from build123d import *

# Parameters (mm, degrees)
F0_R     = 22.03
F1_DEPTH = 50
F2_R     = 5


with BuildPart() as f1:
    # F0 (on Top) → F1 (new body)
    with BuildSketch(Plane.XY):
        with BuildLine():
            ThreePointArc((19.111431778, -6.8960115293), (56.4366245885, -5.6218490797), (74.7410013376, 26.9318496366))
            ThreePointArc((74.7410013376, 26.9318496366), (31.369006979, 64.6653370911), (0, 16.4892914742))
            ThreePointArc((0, 16.4892914742), (7.1396320987, 2.8221168918), (19.111431778, -6.8960115293))
        make_face()
        with Locations((36.6410013376, 26.9318496366)):
            Circle(F0_R, mode=Mode.SUBTRACT)
        with BuildLine():
            ThreePointArc((19.111431778, -6.8960115293), (7.1396320987, 2.8221168918), (0, 16.4892914742))
            Line((0, 16.4892914742), (-34.7932870747, -12.0488790092))
            Line((-34.7932870747, -12.0488790092), (-17.0362032183, -33.6980354112))
            Line((-17.0362032183, -33.6980354112), (19.111431778, -6.8960115293))
        make_face()
    extrude(amount=F1_DEPTH)

    # F2
    f2_edges = [f1.edges().sort_by_distance(p)[0] for p in [
        (66.142371, 51.041582, 50),
        (14.611001, 26.93185, 50),
        (-17.396644, 2.220206, 50),
        (1.037614, -20.297023, 50),
        (0, 16.489291, 25),
        (-34.793287, -12.048879, 25),
        (19.111432, -6.896012, 25),
        (-17.036203, -33.698035, 25),
        (-25.914745, -22.873457, 0),
        (-25.914745, -22.873457, 50),
        (66.142371, 51.041582, 0),
        (14.611001, 26.93185, 0),
        (-17.396644, 2.220206, 0),
        (1.037614, -20.297023, 0),
    ]]
    fillet(f2_edges, radius=F2_R)


solid = f1.part
Can you work these out from the model? Positions are in its coordinate system, mm. Round coordinates to 2 decimals unless told otherwise and drop trailing zeros. Order: outer loops, then holes, each group sorted by start corner. A loop starts at its lowest first (then second) coordinate and runs counter-clockwise, first axis right, second up. Notation, with made-up numbers: (30.5, 38) -> (67.5, 38) arc R26 cw to (67.5, 75) -> close; hole circle Ø8 at (81.25, -18). An arc over 180 degrees is marked (long way). Write each question's results on one line, items separated by ' | '. Start each with the question number.
Item 1: Please list where these lines run through material, in increasing order: L1, parallel to Z at x = 41, y = 0.5; L2, parallel to Y at x = 20, z = 32; L3, parallel to X at y = 15, z = 23.5.
Item 2: Will these pins go through, and if not, where does the flat tip stop? pin 1 (6 mm diameter, centred on x = 0, z = 22, fed in from -Y); pin 2 (1 mm diameter, centred on x = 39.5, y = 52, fed in from -Z); pin 3 (8 mm diameter, centred on y = 6.5, z = 41.5, fed in from +X).
Item 3: If we section it at A-A, the plane z = 32: Write out the boundary of the cut face in (x, y), then the cut area to 3 significant figures.
Item 4: Thinking about a two-plate mould opening in Y: for faces 1 (the cylindrical face through (48.48, 45.51, 24.72)), 2 (the cylindrical face through (-24.656, -22.16, 1.504)), 3 (the flat face through (-16.48, 2.97, 24.72)), which applies, +Y half, -Y half, draft (parallel to the pull), parting line (faces both ways), or undercut?
Results:
1) L1: z = 0.01 to 49.99 | L2: y = -7.7 to 12.5, 41.37 to 61.21 | L3: x = -1.9 to 18.12, 55.16 to 72.82
2) pin 1: stops at y = -23.29 | pin 2: stops at z = 0.17 | pin 3: stops at x = 71.02
3) outline: (-31.62, -15.91) -> (-20.06, -30.02) arc R5 ccw to (-13.21, -30.86) -> (16.71, -8.68) arc R5 cw to (21.65, -8.1) arc R38.1 ccw (long way) to (-0.7, 19.36) arc R5 cw to (-2.43, 14.5) -> (-30.93, -8.88) arc R5 ccw to start; hole circle Ø44.06 at (36.64, 26.93) | area: 4,270 mm2
4) face 1: undercut | face 2: -Y half | face 3: +Y half
